For this review, take the finished solid that the model builds, in its own axes (mm). A direction names the side the tool comes from. Round coordinates to 2 decimals unless told otherwise and drop trailing zeros. Order: outer loops, then holes, each group sorted by start corner. A loop starts at its lowest first (then second) coordinate and runs counter-clockwise, first axis right, second up. Notation, with made-up numbers: (75.25, 79) - (93.25, 79) arc R12 ccw to (93.25, 96) - close; hole circle Ø1 at (16.25, -40). An arc over 180 degrees is marked (long way). One line per item, written item: value.
```python
from build123d import *

# Parameters (mm, degrees)
EXTRUDE_1_DEPTH        = 5
HOLE_WIZARD_M6_1_D     = 5
HOLE_WIZARD_M6_1_DEPTH = 15
HOLE_WIZARD_M6_1_TIP   = 1.502151548


with BuildPart() as part:
    # 草图1 → 凸台-拉伸1 (new, symmetric)
    with BuildSketch(Plane.XY):
        with BuildLine():
            Line((-2.8, 4.7), (2.8, 4.7))
            ThreePointArc((2.8, 4.7), (2.941421356, 4.641421356), (3, 4.5))
            Line((3, 4.5), (3, 3.2))
            Line((3, 3.2), (4.5, 3.2))
            ThreePointArc((4.5, 3.2), (4.641421356, 3.141421356), (4.7, 3))
            Line((4.7, 3), (4.7, 2.45))
            ThreePointArc((4.7, 2.45), (4.047583818, 0.994220712), (2.8, 0))
            Line((2.8, 0), (-2.8, 0))
            ThreePointArc((-2.8, 0), (-4.047583818, 0.994220712), (-4.7, 2.45))
            Line((-4.7, 2.45), (-4.7, 3))
            ThreePointArc((-4.7, 3), (-4.641421356, 3.141421356), (-4.5, 3.2))
            Line((-4.5, 3.2), (-3, 3.2))
            Line((-3, 3.2), (-3, 4.5))
            ThreePointArc((-3, 4.5), (-2.941421356, 4.641421356), (-2.8, 4.7))
        make_face()
    extrude(amount=EXTRUDE_1_DEPTH, both=True)

    # M6 螺纹孔1
    with Locations(Plane.ZX.offset(4.7)):
        with Locations((0, 0)):
            Hole(HOLE_WIZARD_M6_1_D / 2, depth=HOLE_WIZARD_M6_1_DEPTH)
            with Locations((0, 0, -(HOLE_WIZARD_M6_1_DEPTH + HOLE_WIZARD_M6_1_TIP / 2))):  # 118° drill point
                Cone(0, HOLE_WIZARD_M6_1_D / 2, HOLE_WIZARD_M6_1_TIP, mode=Mode.SUBTRACT)


solid = part.part
```
Item 1: Take a section at A-A (z = 0). Write out the cut boundary in (x, y), plus the area to 3 significant figures.
Returned:
outline: (-4.7, 2.45) arc R3.38 ccw to (-2.8, 0) - (-2.5, 0) - (-2.5, 4.7) - (-2.8, 4.7) arc R0.2 ccw to (-3, 4.5) - (-3, 3.2) - (-4.5, 3.2) arc R0.2 ccw to (-4.7, 3) - close; (2.5, 0) - (2.8, 0) arc R3.38 ccw to (4.7, 2.45) - (4.7, 3) arc R0.2 ccw to (4.5, 3.2) - (3, 3.2) - (3, 4.5) arc R0.2 ccw to (2.8, 4.7) - (2.5, 4.7) - close
area: 12.5 mm^2
Item 2: The part is to be moulded in two halves that separate along Z. For faces 1 (the cylindrical face through (-2.44, 2.32, 0.54)), 2 (the flat face through (0, 2, -5)), 3 (the flat face through (-3, 4, 0)), 4 (the flat face through (0, 2, 5)), say which applies: +Z half, -Z half, draft (parallel to the pull), parting line (faces both ways), or undercut.
Returned:
face 1: undercut
face 2: -Z half
face 3: draft
face 4: +Z half
Item 3: Machinability: for faces 5 (the flat face through (4, 3.2, 0)), 6 (the cylindrical face through (4.06, 1.01, 0.07)), 7 (the flat face through (-4, 3.2, 0)), which of the approach directions +Z, -Z, +X, -X, +Y, -Y give a long, thin tool a straight path to every point of the face, cutting with its end or side? Answer none if there is none.
Returned:
face 5: +Z, -Z, +X, +Y
face 6: +Z, -Z, +X, -Y
face 7: +Z, -Z, -X, +Y
Item 4: Wall thickness on line 1 (Z direction, x = -1.5, y = 4.2); line 2 (X direction, y = 4.2, z = 1.5); line 3 (X direction, y = 2.65, z = 0): over which ranges is each line inside the solid? List them lowest first.
Returned:
line 1: -5 to -2, 2 to 5
line 2: -3 to -2, 2 to 3
line 3: -4.7 to -2.5, 2.5 to 4.7
Item 5: Take a section at B-B (x = -1.5). Write out the cut boundary in (y, z), plus the area to 3 significant figures.
Returned:
outline: (0, -5) - (4.7, -5) - (4.7, -2) - (0, -2) - close; (0, 2) - (4.7, 2) - (4.7, 5) - (0, 5) - close
area: 28.2 mm^2
Item 6: Take a section at D-D (y = 3.8). Write out the cut boundary in (x, z), plus the area to 3 significant figures.
Returned:
outline: (-3, -5) - (3, -5) - (3, 5) - (-3, 5) - close; hole circle Ø5 at (0, 0)
area: 40.4 mm^2
Item 7: Take a section at C-C (z = -3.5). Write out the cut boundary in (x, y), plus the area to 3 significant figures.
Returned:
outline: (-4.7, 2.45) arc R3.38 ccw to (-2.8, 0) - (2.8, 0) arc R3.38 ccw to (4.7, 2.45) - (4.7, 3) arc R0.2 ccw to (4.5, 3.2) - (3, 3.2) - (3, 4.5) arc R0.2 ccw to (2.8, 4.7) - (-2.8, 4.7) arc R0.2 ccw to (-3, 4.5) - (-3, 3.2) - (-4.5, 3.2) arc R0.2 ccw to (-4.7, 3) - close
area: 36.0 mm^2
